Read the model definition and answer for the solid it produces. Units are mm, in the model's axes. A direction names the side the tool comes from. Coordinates: 2 decimals unless noted, no trailing zeros. Order: outer loops, then holes, each group sorted by start corner. A loop starts at its lowest first (then second) coordinate and runs counter-clockwise, first axis right, second up. Notation, with made-up numbers: M 76.25,20.25 L 131.25,20.25 A16 ccw 131.25,45.25 Z; hole C 0,23 d9. An arc over 180 degrees is marked long. Use a Markdown table: item, result. Add a question column.
1) Find the intervals of material crossed by probe 1 along Z at (x, y) = (-3.3, 0); probe 2 along Y at (x, z) = (0, 1.05); probe 3 along Z at (x, y) = (-8.5, 57), in increasing order. Write a range as [from, to].
2) Find section C-C on z = 7. Write down the section's boundary in (x, y) (1 decimal), plus the area to 3 significant figures.
3) Find section D-D on y = 20.5. Write down the section's boundary in (x, z), plus the area to 3 significant figures.
4) Find section B-B on x = 0.25. Write down the section's boundary in (y, z), plus the area to 3 significant figures.
5) Find section A-A on y = 60. Write down the section's boundary in (x, z), plus the area to 3 significant figures.
6) The mould has two halves that part along X. Classify faces 4 (the face through (-5.021, -1.584, 4.306)), 5 (the face through (-11.14, 59.11, 1.52)), 6 (the face through (8.014, -9.593, 6.902)): released by +X, released by -X, zero draft, split by the parting line, or undercut.
7) Each of these flat-tipped pins is pushed along its axis until it touches: pin 1 Ø4 at (y, z) = (37.5, 6.5) entering from +X; pin 2 Ø2.5 at (y, z) = (0, 7) entering from -X; pin 3 Ø5 at (x, y) = (0, 60) entering from -Z; pin 4 Ø2.5 at (x, z) = (-5, 10.5) entering from +Y. Where does it stop, or does it pass through?
8) For faces 1 (the face through (-8.64, 48.984, 7.056)), 2 (the face through (-5.02, 1.54, 4.28)), 3 (the face through (-1.77, 14.1, 7.1)), determine the directions among +Z, -Z, +X, -X, +Y, -Y from which every point of the face is accessible in a straight line to the end or side of a thin tool.
from build123d import *

# Parameters (mm, degrees)
CROQUIS1_R              = 3
SALIENTE_EXTRUIR1_DEPTH = 14
REDONDEO1_R             = 10
REDONDEO2_R             = 10
REDONDEO3_R             = 5
CORTAR_EXTRUIR1_START   = -3
CROQUIS2_R              = 14
CORTAR_EXTRUIR1_DEPTH   = 8
CROQUIS3_R              = 1.5
CORTAR_EXTRUIR2_DEPTH   = 10
CROQUIS4_R              = 5
CORTAR_EXTRUIR3_DEPTH   = 3
CORTAR_EXTRUIR4_START   = -3
CROQUIS5_R              = 1.5
CORTAR_EXTRUIR4_DEPTH   = 3


with BuildPart() as part:
    # Croquis1 → Saliente-Extruir1 (new body)
    with BuildSketch(Plane.XY):
        with BuildLine():
            ThreePointArc((-12.5, 0), (9.842509843, -7.705517504), (-3, 12.1346611))
            Line((-3, 12.1346611), (-3, 54.803847577))
            ThreePointArc((-3, 54.803847577), (5.999605182, 59.93116932), (-2.88, 65.263610928))
            Line((-2.88, 65.263610928), (-12.5, 60))
            Line((-12.5, 60), (-12.5, 0))
        make_face()
        Circle(CROQUIS1_R, mode=Mode.SUBTRACT)
        with Locations((0, 60)):
            Circle(CROQUIS1_R, mode=Mode.SUBTRACT)
    extrude(amount=SALIENTE_EXTRUIR1_DEPTH)

    # Redondeo1
    redondeo1_edges = [part.edges().sort_by_distance(p)[0] for p in [
        (-12.5, 60, 7),
    ]]
    fillet(redondeo1_edges, radius=REDONDEO1_R)

    # Redondeo2
    redondeo2_edges = [part.edges().sort_by_distance(p)[0] for p in [
        (-3, 54.803847577, 7),
    ]]
    fillet(redondeo2_edges, radius=REDONDEO2_R)

    # Redondeo3
    redondeo3_edges = [part.edges().sort_by_distance(p)[0] for p in [
        (-3, 12.1346611, 7),
    ]]
    fillet(redondeo3_edges, radius=REDONDEO3_R)

    # Croquis2 → Cortar-Extruir1 (cut)
    with BuildSketch(Plane.XY.offset(14).offset(CORTAR_EXTRUIR1_START)):
        with Locations((0, 60)):
            Circle(CROQUIS2_R)
    extrude(amount=-CORTAR_EXTRUIR1_DEPTH, mode=Mode.SUBTRACT)

    # Croquis3 → Cortar-Extruir2 (cut)
    with BuildSketch(Plane.ZY.offset(12.5)):
        with Locations((7, 0)):
            Circle(CROQUIS3_R)
    extrude(amount=-CORTAR_EXTRUIR2_DEPTH, mode=Mode.SUBTRACT)

    # Croquis4 → Cortar-Extruir3 (cut)
    with BuildSketch(Plane.ZY.offset(12.5)):
        with Locations((7, 0)):
            Circle(CROQUIS4_R)
    extrude(amount=-CORTAR_EXTRUIR3_DEPTH, mode=Mode.SUBTRACT)

    # Croquis5 → Cortar-Extruir4 (cut)
    with BuildSketch(Plane.ZY.offset(9.5).offset(CORTAR_EXTRUIR4_START)):
        Polygon((8.804219591, 3.125), (8.804219591, -3.125), (5.195780409, -3.125), (3.391560818, 0), (5.195780409, 3.125), align=None)
        with Locations((7, 0)):
            Circle(CROQUIS5_R, mode=Mode.SUBTRACT)
        Polygon((10.608439182, 0), (8.804219591, 3.125), (8.804219591, -3.125), align=None)
        with BuildLine():
            Line((8.804219591, 3.125), (10.608439182, 0))
            Line((10.608439182, 0), (8.804219591, -3.125))
            Line((8.804219591, -3.125), (10.903123749, -3.125))
            ThreePointArc((10.903123749, -3.125), (11.717818285, -1.655956107), (12, 0))
            ThreePointArc((12, 0), (11.717818285, 1.655956107), (10.903123749, 3.125))
            Line((10.903123749, 3.125), (8.804219591, 3.125))
        make_face()
        with BuildLine():
            Line((14, 3.125), (10.903123749, 3.125))
            ThreePointArc((10.903123749, 3.125), (11.717818285, 1.655956107), (12, 0))
            ThreePointArc((12, 0), (11.717818285, -1.655956107), (10.903123749, -3.125))
            Line((10.903123749, -3.125), (14, -3.125))
            Line((14, -3.125), (14, 3.125))
        make_face()
    extrude(amount=-CORTAR_EXTRUIR4_DEPTH, mode=Mode.SUBTRACT)


solid = part.part
Check result:
| question | item | result |
|---|---|---|
| 1 | probe 1 | z = [0, 5.5], [8.5, 14] |
| 1 | probe 2 | y = [-12.5, -3], [3, 12.8], [52.75, 57], [63, 66] |
| 1 | probe 3 | z = [0, 3], [11, 14] |
| 2 | outline | M -12.5,5 L -9.5,5 L -9.5,1.5 L -6.5,1.5 L -6.5,3.1 L -3.5,3.1 L -3.5,1.5 L -2.6,1.5 A3 cw long -2.6,-1.5 L -3.5,-1.5 L -3.5,-3.1 L -6.5,-3.1 L -6.5,-1.5 L -9.5,-1.5 L -9.5,-5 L -11.5,-5 A12.5 ccw long 1.4,12.4 A5 cw -3,17.4 L -3,45.6 A10 cw -3,46.3 A14 cw -12.5,53.7 Z |
| 2 | area | 788 mm2 |
| 3 | outline | M -12.5,0 L -3,0 L -3,14 L -12.5,14 Z |
| 3 | area | 133 mm2 |
| 4 | outline | M -12.5,0 L -2.99,0 L -2.99,14 L -12.5,14 Z; M 2.99,0 L 12.7,0 L 12.7,14 L 2.99,14 Z; M 52.99,0 L 57.01,0 L 57.01,3 L 52.99,3 Z; M 52.99,11 L 57.01,11 L 57.01,14 L 52.99,14 Z; M 62.99,0 L 65.99,0 L 65.99,3 L 62.99,3 Z; M 62.99,11 L 65.99,11 L 65.99,14 L 62.99,14 Z |
| 4 | area | 311 mm2 |
| 5 | outline | M -10.55,0 L -3,0 L -3,3 L -10.55,3 Z; M -10.55,11 L -3,11 L -3,14 L -10.55,14 Z; M 3,0 L 6,0 L 6,3 L 3,3 Z; M 3,11 L 6,11 L 6,14 L 3,14 Z |
| 5 | area | 63.3 mm2 |
| 6 | face 4 | undercut |
| 6 | face 5 | released by -X |
| 6 | face 6 | split by the parting line |
| 7 | pin 1 | stops at x = -3 |
| 7 | pin 2 | stops at x = 2.73 |
| 7 | pin 3 | passes through |
| 7 | pin 4 | stops at y = 64.73 |
| 8 | face 1 | +X, +Y |
| 8 | face 2 | +Z |
| 8 | face 3 | +Z, -Z, +X |
